from build123d import *

# Parameters (mm, degrees)
SKETCH1_R           = 1.6
BOSS_EXTRUDE1_DEPTH = 4
FILLET1_R           = 5


with BuildPart() as part:
    # Sketch1 → Boss-Extrude1 (new body)
    with BuildSketch(Plane.XY):
        with BuildLine():
            Line((20, 32), (-25, 32))
            Line((-25, 32), (-25, -10))
            Line((-25, -10), (-0.78093138, -10))
            ThreePointArc((-0.78093138, -10), (-0.832904243, -9.966038414), (-0.882669446, -9.928917093))
            ThreePointArc((-0.882669446, -9.928917093), (-0.231731966, -8.146704874), (0.316845382, -9.963037138))
            ThreePointArc((0.316845382, -9.963037138), (0.289034097, -9.981991883), (0.260600707, -10))
            Line((0.260600707, -10), (20, -10))
            Line((20, -10), (20, 32))
        make_face()
        with Locations((-20, 7.45)):
            Circle(SKETCH1_R, mode=Mode.SUBTRACT)
        with BuildLine():
            ThreePointArc((5.442708333, -2.641860329), (-6.05, 0), (5.442708333, 2.641860329))
            ThreePointArc((5.442708333, 2.641860329), (8.7, 0), (5.442708333, -2.641860329))
        make_face(mode=Mode.SUBTRACT)
        with Locations((-20, 19.45)):
            Circle(SKETCH1_R, mode=Mode.SUBTRACT)
        with BuildLine():
            ThreePointArc((1.25114395, 18.628974283), (-0.217290022, 18.701098604), (-0.026825007, 20.158913176))
            ThreePointArc((-0.026825007, 20.158913176), (0.578619081, 20.341772292), (1.172689821, 20.124793131))
            ThreePointArc((1.172689821, 20.124793131), (1.548813096, 19.39455356), (1.25114395, 18.628974283))
        make_face(mode=Mode.SUBTRACT)
        with Locations((0, 26.9)):
            Circle(SKETCH1_R, mode=Mode.SUBTRACT)
    extrude(amount=BOSS_EXTRUDE1_DEPTH)

    # Fillet1
    fillet1_edges = [part.edges().sort_by_distance(p)[0] for p in [
        (-25, -10, 2),
        (-25, 32, 2),
        (20, 32, 2),
        (20, -10, 2),
    ]]
    fillet(fillet1_edges, radius=FILLET1_R)


solid = part.part
Work out the finished part from the listing and answer in its coordinate system (mm). Coordinates: 2 decimals unless noted, no trailing zeros. Loops run counter-clockwise (first coordinate to the right, second up) from the corner with the lowest first, then second, coordinate; pieces in that order, holes last. Notation, with made-up numbers: (42, -15.5) -> (60, -15.5) arc R12 cw to (60, 7.5) -> close; hole circle Ø1 at (51, -10.75). An arc over 180 degrees is marked (long way). Write each question's results on one line, items separated by ' | '. Start each with the question number.
1) Find section D-D on z = 2.45. Determine the outline of the cut face in (x, y).
2) The mould has two halves that part along X. Classify faces 1 (the flat face through (-2, 32, 2)), 2 (the cylindrical face through (-21.27, 6.48, 1.97)), 3 (the cylindrical face through (-23, 31, 2)), 4 (the cylindrical face through (-6.046, -0.228, 1.972)): pulls with the +X half, pulls with the -X half, needs draft (parallel to the pull), parting line crosses it, or undercut.
3) Find section C-C on y = 19.45. Determine the outline of the cut face in (x, z).
4) Find section B-B on x = 6. Determine the outline of the cut face in (y, z), then the cut area to 3 significant figures.
5) Find section A-A on y = 0. Determine the outline of the cut face in (x, z), then the cut area to 3 significant figures.
6) Consider line 1 along Y through (x, z) = (-20.5, 2.45); line 2 along Y through (x, z) = (0.5, 0.75); line 3 along X through (y, z) = (0, 2.85). Determine where each line is inside the solid, lowest interval first.
Response values:
1) outline: (-25, -5) arc R5 ccw to (-20, -10) -> (-0.78, -10) arc R1 cw (long way) to (0.32, -9.96) arc R1 cw to (0.26, -10) -> (15, -10) arc R5 ccw to (20, -5) -> (20, 27) arc R5 ccw to (15, 32) -> (-20, 32) arc R5 ccw to (-25, 27) -> close; hole circle Ø3.2 at (-20, 7.45); hole circle Ø3.2 at (-20, 19.45); hole circle Ø3.2 at (0, 26.9); hole circle Ø2 at (0.55, 19.34); hole (5.44, -2.64) arc R2.7 ccw (long way) to (5.44, 2.64) arc R6.05 ccw (long way) to start
2) face 1: needs draft | face 2: undercut | face 3: pulls with the -X half | face 4: undercut
3) outline: (-25, 0) -> (-21.6, 0) -> (-21.6, 4) -> (-25, 4) -> close; (-18.4, 0) -> (-0.44, 0) -> (-0.44, 4) -> (-18.4, 4) -> close; (1.54, 0) -> (20, 0) -> (20, 4) -> (1.54, 4) -> close
4) outline: (-10, 0) -> (-2.7, 0) -> (-2.7, 4) -> (-10, 4) -> close; (2.7, 0) -> (32, 0) -> (32, 4) -> (2.7, 4) -> close | area: 146 mm^2
5) outline: (-25, 0) -> (-6.05, 0) -> (-6.05, 4) -> (-25, 4) -> close; (8.7, 0) -> (20, 0) -> (20, 4) -> (8.7, 4) -> close | area: 121 mm^2
6) line 1: y = -9.97 to 5.93, 8.97 to 17.93, 20.97 to 31.97 | line 2: y = -10 to -9.8, -8.5 to -6.03, 6.03 to 18.34, 20.34 to 25.38, 28.42 to 32 | line 3: x = -25 to -6.05, 8.7 to 20
